```python
from build123d import *

# Parameters (mm, degrees)
F0_R          = 152.4
F1_DEPTH      = 12.7
F1_DEPTH_BACK = 12.7
F2_R          = 3.858191
F2_R_2        = 1.5875
F3_DEPTH      = 25.4
F5_DEPTH      = 25.401
F6_W          = 0.887787
F6_H          = 5.147254
F7_DEPTH      = 25.4
F8_R          = 6.462154
F8_R_2        = 3.194713
F9_DEPTH      = 6.985


with BuildPart() as f1:
    # F0 (on Top) → F1 (new body, two sides)
    with BuildSketch(Plane.XY) as f1_sk:
        Circle(F0_R)
    extrude(amount=F1_DEPTH)
    extrude(f1_sk.sketch, amount=-F1_DEPTH_BACK)

    # F2 (on face) → F3 (join)
    with BuildSketch(Plane.XY.offset(12.7)):
        Circle(F2_R)
        Circle(F2_R_2, mode=Mode.SUBTRACT)
    extrude(amount=F3_DEPTH)

    # F4 (on face) → F5 (cut, through all)
    with BuildSketch(Plane.XY.offset(12.7)):
        with BuildLine():
            Line((-20.428086, -19.901165), (-129.102567, -19.901165))
            ThreePointArc((-129.102567, -19.901165), (-92.555914, -92.178804), (-20.428086, -129.02024))
            Line((-20.428086, -129.02024), (-20.428086, -19.901165))
        make_face()
        with BuildLine():
            Line((-129.102567, 19.901165), (-20.428086, 19.901165))
            Line((-20.428086, 19.901165), (-20.428086, 129.02024))
            ThreePointArc((-20.428086, 129.02024), (-92.555914, 92.178804), (-129.102567, 19.901165))
        make_face()
        with BuildLine():
            Line((20.428086, 129.02024), (20.428086, 19.901165))
            Line((20.428086, 19.901165), (129.102567, 19.901165))
            ThreePointArc((129.102567, 19.901165), (92.555914, 92.178804), (20.428086, 129.02024))
        make_face()
        with BuildLine():
            ThreePointArc((20.428086, -129.02024), (92.555914, -92.178804), (129.102567, -19.901165))
            Line((129.102567, -19.901165), (20.428086, -19.901165))
            Line((20.428086, -19.901165), (20.428086, -129.02024))
        make_face()
    extrude(amount=-F5_DEPTH, mode=Mode.SUBTRACT)

    # F6 (on face) → F7 (join)
    with BuildSketch(Plane.XY.offset(12.7)):
        with Locations((1.491769, -0.241479)):
            Rectangle(F6_W, F6_H)
    extrude(amount=F7_DEPTH)

    # F8 (on face) → F9 (join)
    with BuildSketch(Plane(origin=(0, 0, -12.7), x_dir=(1, 0, 0), z_dir=(0, 0, -1))):
        Circle(F8_R)
        Circle(F8_R_2, mode=Mode.SUBTRACT)
    extrude(amount=F9_DEPTH)


solid = f1.part
```
Input: part model. Units: mm. Frame: model coordinates. A direction names the side the tool comes from. Give positions to 0.01 mm unless a question says otherwise; leave off trailing zeros. Loops run counter-clockwise (first coordinate to the right, second up) from the corner with the lowest first, then second, coordinate; pieces in that order, holes last.
1) Line query: L1, parallel to Y at x = 72.5, z = 6.5; L2, parallel to Y at x = -93, z = -2.5; L3, parallel to X at y = -32.5, z = -8.5. Output: solid intervals per line, ascending.
A:
L1: y = -134.05 to -108.66, -19.9 to 19.9, 108.66 to 134.05
L2: y = -120.73 to -91.73, -19.9 to 19.9, 91.73 to 120.73
L3: x = -148.89 to -126.52, -20.43 to 20.43, 126.52 to 148.89
2) Section query C-C on z = 19. Return the cut outline in (x, y) (1 decimal).
A:
outline: circle Ø7.7 at (0, 0); hole (1, -1.2) - (1, 1.2) arc R1.6 ccw (long way) to start
3) Mould query, pull axis Y, two halves, no side actions, for faces 4 (the flat face through (2, 0, 38.1)), 5 (the flat face through (-20.428, -75, 0)), 6 (the cylindrical face through (-1.4, 6.31, -16.14)), 7 (the flat face through (-76, 19.901, 0)). Classes: released by +Y, released by -Y, zero draft, split by the parting line, or undercut.
A:
face 4: zero draft
face 5: undercut
face 6: split by the parting line
face 7: undercut
4) Contact query for flat-ended pins moving along their axis: pin 1 (2 mm diameter, centred on y = -96, z = -10, fed in from +X); pin 2 (20.5 mm diameter, centred on x = 94, z = -2, fed in from +Y); pin 3 (7 mm diameter, centred on x = -1, y = 0.5, fed in from -Z) (3 decimals); pin 4 (3 mm diameter, centred on y = -10.5, z = 4, fed in from +X). Output: stop coordinate, or through.
A:
pin 1: stops at x = 119.17
pin 2: stops at y = 127.33
pin 3: stops at z = -19.685
pin 4: stops at x = 152.13
5) Section query B-B on y = -88. Return the cut outline in (x, z), and give its area (3 significant figures).
A:
outline: (-124.43, -12.7) - (-96.54, -12.7) - (-96.54, 12.7) - (-124.43, 12.7) - close; (-20.43, -12.7) - (20.43, -12.7) - (20.43, 12.7) - (-20.43, 12.7) - close; (96.54, -12.7) - (124.43, -12.7) - (124.43, 12.7) - (96.54, 12.7) - close
area: 2,450 mm2
6) Reachability of faces 1 (the flat face through (20.428, 75, 0)), 2 (the cylindrical face through (-3.1, -2.3, 25.2)), 3 (the flat face through (32, 2, -12.7)) from +Z, -Z, +X, -X, +Y, -Y: full face, straight path, thin tool, end or side. Return the list, or none.
A:
face 1: +Z, -Z
face 2: +Z
face 3: -Z
7) Section query A-A on x = -86. Return the cut outline in (y, z).
A:
outline: (-125.82, -12.7) - (-98.32, -12.7) - (-98.32, 12.7) - (-125.82, 12.7) - close; (-19.9, -12.7) - (19.9, -12.7) - (19.9, 12.7) - (-19.9, 12.7) - close; (98.32, -12.7) - (125.82, -12.7) - (125.82, 12.7) - (98.32, 12.7) - close
